Work out the finished part from the listing and answer in its coordinate system (mm). Face numbers are marked on the shaded views. Round coordinates to 2 decimals unless told otherwise and drop trailing zeros. Loops run counter-clockwise (first coordinate to the right, second up) from the corner with the lowest first, then second, coordinate; pieces in that order, holes last. Notation, with made-up numbers: (56, 37) -> (78, 37) arc R27 ccw to (78, 71) -> close; hole circle Ø1 at (35, 42.5). An arc over 180 degrees is marked (long way). Write item = value, one per line. Start each with the question number.
```python
from build123d import *

# Parameters (mm, degrees)
SKETCH1_W           = 22.5
SKETCH1_H           = 60
BOSS_EXTRUDE1_DEPTH = 4.5
CUT_EXTRUDE3_DEPTH  = 1.6
FILLET1_R           = 1
CUT_EXTRUDE4_START  = -1.9
SKETCH5_R           = 2.3
CUT_EXTRUDE4_DEPTH  = 1.9
SKETCH6_R           = 1.05
CUT_EXTRUDE5_DEPTH  = 1
BOSS_EXTRUDE2_DEPTH = 4.5
CUT_EXTRUDE6_DEPTH  = 4.5
SKETCH11_R          = 4.875
CUT_EXTRUDE8_DEPTH  = 4.5
CUT_EXTRUDE9_DEPTH  = 4.5
FILLET2_R           = 7.5
FILLET3_R           = 7.5


with BuildPart() as part:
    # Sketch1 → Boss-Extrude1 (new body)
    with BuildSketch(Plane(origin=(0, 0, 0), x_dir=(1, 0, 0), z_dir=(0, 1, 0))):
        Rectangle(SKETCH1_W, SKETCH1_H)
    extrude(amount=BOSS_EXTRUDE1_DEPTH)

    # Sketch4 → Cut-Extrude3 (cut)
    with BuildSketch(Plane(origin=(-18.455631439, 0, 11.83964206), x_dir=(0, 0, -1), z_dir=(0, -1, 0))):
        with BuildLine():
            Line((4.08964206, 21.947970461), (18.28964206, 20.705631439))
            ThreePointArc((18.28964206, 20.705631439), (20.53964206, 18.455631439), (18.28964206, 16.205631439))
            Line((18.28964206, 16.205631439), (4.08964206, 14.963292417))
            Line((4.08964206, 14.963292417), (4.08964206, 11.213292417))
            ThreePointArc((4.08964206, 11.213292417), (1.83964206, 8.963292417), (-0.41035794, 11.213292417))
            Line((-0.41035794, 11.213292417), (-0.41035794, 15.17326521))
            Line((-0.41035794, 15.17326521), (-12.21035794, 16.205631439))
            ThreePointArc((-12.21035794, 16.205631439), (-14.46035794, 18.455631439), (-12.21035794, 20.705631439))
            Line((-12.21035794, 20.705631439), (-0.41035794, 21.737997669))
            Line((-0.41035794, 21.737997669), (-0.41035794, 25.697970461))
            ThreePointArc((-0.41035794, 25.697970461), (1.83964206, 27.947970461), (4.08964206, 25.697970461))
            Line((4.08964206, 25.697970461), (4.08964206, 21.947970461))
        make_face()
    extrude(amount=-CUT_EXTRUDE3_DEPTH, mode=Mode.SUBTRACT)

    # Fillet1
    fillet1_edges = [part.edges().sort_by_distance(p)[0] for p in [
        (3.492339022, 0.8, 7.75),
        (-3.492339022, 0.8, 7.75),
        (-3.28236623, 0.8, 12.25),
        (3.28236623, 0.8, 12.25),
    ]]
    fillet(fillet1_edges, radius=FILLET1_R)

    # Sketch5 → Cut-Extrude4 (cut)
    with BuildSketch(Plane(origin=(0, 4.5, 0), x_dir=(1, 0, 0), z_dir=(0, 1, 0)).offset(CUT_EXTRUDE4_START)):
        with Locations(Location((0, -10, 0), (0, 0, 270))):
            Circle(SKETCH5_R)
    extrude(amount=CUT_EXTRUDE4_DEPTH, mode=Mode.SUBTRACT)

    # Sketch6 → Cut-Extrude5 (cut)
    with BuildSketch(Plane(origin=(0, 2.6, 0), x_dir=(-1, 0, 0), z_dir=(0, -1, 0))):
        with Locations(Location((0, -10, 0), (0, 0, 90))):
            Circle(SKETCH6_R)
    extrude(amount=CUT_EXTRUDE5_DEPTH, mode=Mode.SUBTRACT)

    # Sketch9 → Boss-Extrude2 (add)
    with BuildSketch(Plane(origin=(0, 4.5, 0), x_dir=(1, 0, 0), z_dir=(0, 1, 0))):
        with BuildLine():
            Line((-48.75, -30), (-11.25, -30))
            Line((-11.25, -30), (-11.25, 25.621488653))
            ThreePointArc((-11.25, 25.621488653), (-38.499371855, 3.541019662), (-48.75, -30))
        make_face()
    extrude(amount=-BOSS_EXTRUDE2_DEPTH)

    # Sketch10 → Cut-Extrude6 (cut)
    with BuildSketch(Plane(origin=(0, 4.5, 0), x_dir=(1, 0, 0), z_dir=(0, 1, 0))):
        with BuildLine():
            ThreePointArc((-11.25, 25.621488653), (-0.211035747, 28.89520065), (11.25, 30))
            Line((11.25, 30), (-11.25, 30))
            Line((-11.25, 30), (-11.25, 25.621488653))
        make_face()
    extrude(amount=-CUT_EXTRUDE6_DEPTH, mode=Mode.SUBTRACT)

    # Sketch11 → Cut-Extrude8 (cut)
    with BuildSketch(Plane(origin=(0, 4.5, 0), x_dir=(1, 0, 0), z_dir=(0, 1, 0))):
        with Locations(Location((0, 20, 0), (0, 0, 270))):
            Circle(SKETCH11_R)
    extrude(amount=-CUT_EXTRUDE8_DEPTH, mode=Mode.SUBTRACT)

    # Sketch12 → Cut-Extrude9 (cut)
    with BuildSketch(Plane(origin=(0, 4.5, 0), x_dir=(1, 0, 0), z_dir=(0, 1, 0))):
        with BuildLine():
            Line((-11.25, 1), (-40.121198156, 1))
            ThreePointArc((-40.121198156, 1), (-46.552560018, -13.910747211), (-48.75, -30))
            Line((-48.75, -30), (-11.25, -30))
            Line((-11.25, -30), (-11.25, 1))
        make_face()
    extrude(amount=-CUT_EXTRUDE9_DEPTH, mode=Mode.SUBTRACT)

    # Fillet2
    fillet2_edges = [part.edges().sort_by_distance(p)[0] for p in [
        (-40.121198156, 2.25, -1),
    ]]
    fillet(fillet2_edges, radius=FILLET2_R)

    # Fillet3
    fillet3_edges = [part.edges().sort_by_distance(p)[0] for p in [
        (-11.25, 2.25, 30),
        (11.25, 2.25, 30),
        (11.25, 2.25, -30),
    ]]
    fillet(fillet3_edges, radius=FILLET3_R)


solid = part.part
```
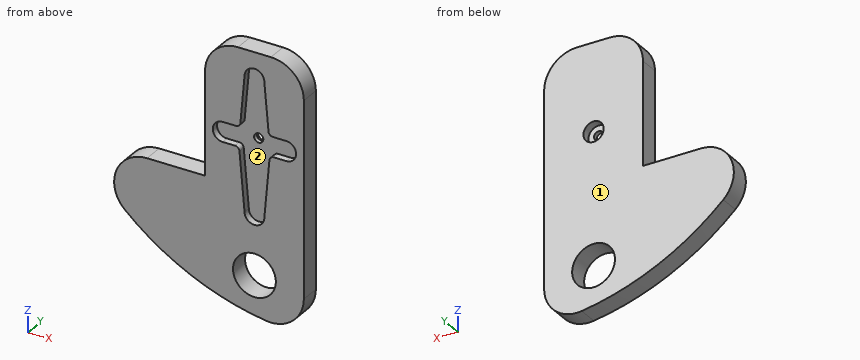
Item 1: Flat-ended cylindrical pins translate along their axes: pin 1 (0.8 mm diameter, centred on x = -5.5, y = 1, fed in from +Z); pin 2 (0.8 mm diameter, centred on x = -5.5, y = 1, fed in from -Z); pin 3 (0.8 mm diameter, centred on x = 6, y = 0.5, fed in from +Z). Find the tip coordinate at first contact, or state that the pin passes through.
Item 2: Find the intervals of material crossed by line 1 along X through (y, z) = (2.25, 10); line 2 along X through (y, z) = (3.35, 9.5) (3 decimals); line 3 along Z through (x, y) = (-4, 1.1), in increasing order. Write a range as [from, to].
Item 3: Section D-D (z = -20) is taken. Determine the outline of the cut face in (x, y) (3 decimals), then the cut area to 3 significant figures.
Item 4: Section C-C (x = 0) is taken. Determine the outline of the cut face in (y, z) (3 decimals).
Item 5: Section B-B (y = 3.85) is taken. Determine the outline of the cut face in (x, z) (3 decimals), then the cut area to 3 significant figures.
Item 6: Section A-A (z = 10) is taken. Determine the outline of the cut face in (x, y), then the cut area to 3 significant figures.
Item 7: The mould has two halves that part along Z. Classify the marked faces 1 and 2: pulls with the +Z half, pulls with the -Z half, needs draft (parallel to the pull), parting line crosses it, or undercut.
Worked answers:
q1.pin_1 = 29.88
q1.pin_2 = -27.73
q1.pin_3 = 29.77
q2.line_1 = [-11.25, -1.05], [1.05, 11.25]
q2.line_2 = [-11.25, -2.245], [2.245, 11.25]
q2.line_3 = [-28.03, -22.79], [-17.21, 7.66], [12.27, 30]
q3.outline = (-21.916, 0) -> (-4.875, 0) -> (-4.875, 4.5) -> (-21.916, 4.5) -> close; (4.875, 0) -> (11.25, 0) -> (11.25, 4.5) -> (4.875, 4.5) -> close
q3.area = 105 mm2
q4.outline = (0, -28.936) -> (4.5, -28.936) -> (4.5, -24.875) -> (0, -24.875) -> close; (0, -15.125) -> (4.5, -15.125) -> (4.5, 7.7) -> (2.6, 7.7) -> (2.6, 8.95) -> (1.6, 8.95) -> (1.6, -8.7) -> (0, -8.7) -> close; (0, 26.3) -> (1.6, 26.3) -> (1.6, 11.05) -> (2.6, 11.05) -> (2.6, 12.3) -> (4.5, 12.3) -> (4.5, 30) -> (0, 30) -> close
q5.outline = (-29.542, -14) arc R60 ccw to (2.679, -29.385) arc R7.5 ccw to (11.25, -21.962) -> (11.25, 22.5) arc R7.5 ccw to (3.75, 30) -> (-3.75, 30) arc R7.5 ccw to (-11.25, 22.5) -> (-11.25, -1) -> (-24.443, -1) arc R7.5 ccw to start; hole circle Ø9.75 at (0, -20); hole circle Ø4.6 at (0, 10)
q5.area = 1,560 mm2
q6.outline = (-11.25, 0) -> (-9.49, 0) -> (-9.49, 1.6) -> (-1.05, 1.6) -> (-1.05, 2.6) -> (-2.3, 2.6) -> (-2.3, 4.5) -> (-11.25, 4.5) -> close; (1.05, 1.6) -> (9.49, 1.6) -> (9.49, 0) -> (11.25, 0) -> (11.25, 4.5) -> (2.3, 4.5) -> (2.3, 2.6) -> (1.05, 2.6) -> close
q6.area = 60.0 mm2
q7.face_1 = needs draft
q7.face_2 = undercut
